Check sheet for the modelled part. Datum: model origin and axes. Units: mm. A direction names the side the tool comes from. Give positions to 0.01 mm unless a question says otherwise; leave off trailing zeros. Order: outer loops, then holes, each group sorted by start corner. A loop starts at its lowest first (then second) coordinate and runs counter-clockwise, first axis right, second up. Notation, with made-up numbers: (-4, -30.75) -> (18, -30.75) arc R7 ccw to (18, -19.75) -> close; hole circle Ø7 at (12, -40). An arc over 180 degrees is marked (long way). Answer in a Markdown table with one row per item. Add a question column.
(1) Release check for a two-part mould opening along X. For faces 4 (the face through (25, 3, -28)), 5 (the face through (30, 3, -15)), 6 (the face through (8, -20, -28.4)) record: released by +X, released by -X, zero draft, split by the parting line, or undercut.
(2) Go/stop test with flat-tipped pins: pin 1 (2 mm diameter, centred on x = 1.5, y = 6, fed in from -Z); pin 2 (2 mm diameter, centred on y = -3, z = -29, fed in from -X); pin 3 (14.5 mm diameter, centred on x = 13.5, z = -17.5, fed in from +Y). Record where each tip stops, or that it passes through.
(3) Cross-section at B-B (x = 10.5). Record the cut outline in (y, z).
(4) Thickness scan on L1, parallel to Z at x = 12.5, y = -198; L2, parallel to X at y = 16, z = -10; L3, parallel to X at y = 190, z = -26.5. Record the ranges inside material, lowest first. Write a range as [from, to].
(5) Set-up check for faces 1 (the face through (2, 3, -10)), 2 (the face through (8, 20, -28.4)), 3 (the face through (1, 245, -15)): record each of +Z, -Z, +X, -X, +Y, -Y from which the full face is reachable in a straight line by a thin tool's end or side.
(6) Cross-section at A-A (z = -19). Record the cut outline in (x, y).
(7) Cross-section at C-C (y = -59.5). Record the cut outline in (x, z).
```python
from build123d import *

# Parameters (mm, degrees)
EXTRUDE_1_DEPTH     = 245
SKETCH_2_W          = 23
SKETCH_2_H          = 40
CUT_EXTRUDE_1_DEPTH = 18


with BuildPart() as part:
    # 草图1 → 凸台-拉伸1 (new, symmetric)
    with BuildSketch(Plane(origin=(0, 0, 0), x_dir=(1, 0, 0), z_dir=(0, 1, 0))):
        with BuildLine():
            Line((4, 0), (26, 0))
            ThreePointArc((26, 0), (28.828427125, 1.171572875), (30, 4))
            Line((30, 4), (30, 26))
            ThreePointArc((30, 26), (28.828427125, 28.828427125), (26, 30))
            Line((26, 30), (4, 30))
            ThreePointArc((4, 30), (1.171572875, 28.828427125), (0, 26))
            Line((0, 26), (0, 4))
            ThreePointArc((0, 4), (1.171572875, 1.171572875), (4, 0))
        make_face()
        with BuildLine():
            Line((4, 2), (26, 2))
            ThreePointArc((26, 2), (27.414213562, 2.585786438), (28, 4))
            Line((28, 4), (28, 26))
            ThreePointArc((28, 26), (27.414213562, 27.414213562), (26, 28))
            Line((26, 28), (4, 28))
            ThreePointArc((4, 28), (2.585786438, 27.414213562), (2, 26))
            Line((2, 26), (2, 4))
            ThreePointArc((2, 4), (2.585786438, 2.585786438), (4, 2))
        make_face(mode=Mode.SUBTRACT)
    extrude(amount=EXTRUDE_1_DEPTH, both=True)

    # 草图2 → 切除-拉伸1 (cut)
    with BuildSketch(Plane.XY.offset(-30)):
        with Locations((11.5, 0)):
            Rectangle(SKETCH_2_W, SKETCH_2_H)
    extrude(amount=CUT_EXTRUDE_1_DEPTH, mode=Mode.SUBTRACT)


solid = part.part
```
Answer below:
| question | item | result |
|---|---|---|
| 1 | face 4 | undercut |
| 1 | face 5 | released by +X |
| 1 | face 6 | zero draft |
| 2 | pin 1 | stops at z = -12 |
| 2 | pin 2 | stops at x = 23 |
| 2 | pin 3 | passes through |
| 3 | outline | (-245, -30) -> (-20, -30) -> (-20, -28) -> (-245, -28) -> close; (-245, -2) -> (245, -2) -> (245, 0) -> (-245, 0) -> close; (20, -30) -> (245, -30) -> (245, -28) -> (20, -28) -> close |
| 4 | L1 | z = [-30, -28], [-2, 0] |
| 4 | L2 | x = [0, 2], [28, 30] |
| 4 | L3 | x = [0.03, 2.06], [27.94, 29.97] |
| 5 | face 1 | +Y, -Y |
| 5 | face 2 | -Z, -X |
| 5 | face 3 | +Z, -Z, +X, -X, +Y |
| 6 | outline | (0, -245) -> (2, -245) -> (2, -20) -> (0, -20) -> close; (0, 20) -> (2, 20) -> (2, 245) -> (0, 245) -> close; (28, -245) -> (30, -245) -> (30, 245) -> (28, 245) -> close |
| 7 | outline | (0, -26) arc R4 ccw to (4, -30) -> (26, -30) arc R4 ccw to (30, -26) -> (30, -4) arc R4 ccw to (26, 0) -> (4, 0) arc R4 ccw to (0, -4) -> close; hole (2, -26) arc R2 ccw to (4, -28) -> (26, -28) arc R2 ccw to (28, -26) -> (28, -4) arc R2 ccw to (26, -2) -> (4, -2) arc R2 ccw to (2, -4) -> close |
